Job drawing, mm, ordinate dimensions from the low corner. One solid piece. A direction names the side the tool comes from. Coordinates: 2 decimals unless noted, no trailing zeros. Order: outer loops, then holes, each group sorted by start corner. A loop starts at its lowest first (then second) coordinate and runs counter-clockwise, first axis right, second up. Notation, with made-up numbers: (19, -35.75) -> (56, -35.75) arc R34 cw to (56, 0.25) -> close; hole circle Ø9 at (-37.75, 1.25). An arc over 180 degrees is marked (long way). Use CSV: the item, a comma, the result in double quotes. Start each with the question number.
(1) Tool access for the marked faces 1, 2 and 3: list every direction of +Z, -Z, +X, -X, +Y, -Y with a clear straight run to the whole face (end or side of a thin tool).
(2) Cut at B-B on z = 8. Write the cut outline in (x, y).
(3) Cut at D-D on z = 11. Write the cut outline in (x, y), plus the area to 3 significant figures.
(4) Cut at C-C on x = 33. Write the cut outline in (y, z).
(5) Probe L1, parallel to X at y = 1.5, z = 10.5; L2, parallel to Z at x = 10.5, y = 1.75; L3, parallel to Y at x = 23, z = 14. List the from-to ranges inside material, lowest first.
(6) Cut at A-A on y = 6. Write the cut outline in (x, z), plus the area to 3 significant figures.
(7) Pin check, flat tips, straight feed: pin 1 Ø1.9 at (x, z) = (32.5, 8) entering from +Y; pin 2 Ø4 at (y, z) = (8, 2.5) entering from +X. Stop position of each tip, or through.
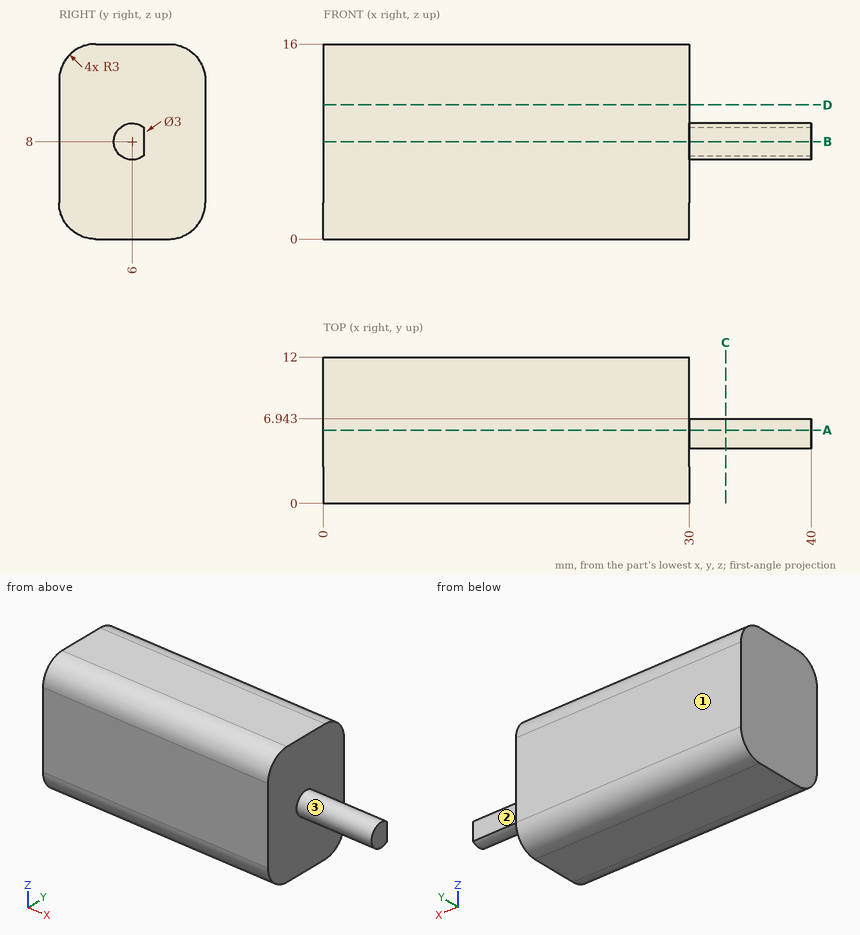
Outcome:
1,face 1,"+Z, -Z, +X, -X, +Y"
1,face 2,"+Z, -Z, +X, +Y"
1,face 3,"+X"
2,outline,"(0, 0) -> (30, 0) -> (30, 4.5) -> (40, 4.5) -> (40, 6.94) -> (30, 6.94) -> (30, 12) -> (0, 12) -> close"
3,outline,"(0, 0) -> (30, 0) -> (30, 12) -> (0, 12) -> close"
3,area,"360 mm2"
4,outline,"(6.94, 6.83) -> (6.94, 9.17) arc R1.5 ccw (long way) to start"
5,L1,"0 to 30"
5,L2,"0.27 to 15.73"
5,L3,"0.17 to 11.83"
6,outline,"(0, 0) -> (30, 0) -> (30, 6.5) -> (40, 6.5) -> (40, 9.5) -> (30, 9.5) -> (30, 16) -> (0, 16) -> close"
6,area,"510 mm2"
7,pin 1,"y = 6.94"
7,pin 2,"x = 30"
